Could you check a few things on this model? Use its own coordinates, in mm. Face numbers are marked on the shaded views. A direction names the side the tool comes from. Give positions to 0.01 mm unless a question says otherwise; leave off trailing zeros. Write each loop counter-clockwise with the first axis right and the second up, starting at its lowest first coordinate (ties: lowest second). Pieces come first, ordered by that corner, then holes. Notation, with made-up numbers: (88.5, -26.75) - (122.5, -26.75) arc R21 cw to (122.5, 7.25) - close; hole circle Ø11 at (-40, 57.25). An arc over 180 degrees is marked (long way). Write item = value, one per line.
from build123d import *

# Parameters (mm, degrees)
BOSS_EXTRUDE1_DEPTH = 4
CUT_EXTRUDE2_DEPTH  = 3.25
SKETCH5_W           = 9.5
SKETCH5_H           = 5
BOSS_EXTRUDE2_DEPTH = 8
SKETCH6_W           = 9.5
SKETCH6_H           = 20
BOSS_EXTRUDE3_DEPTH = 3


with BuildPart() as part:
    # Sketch1 → Boss-Extrude1 (new body)
    with BuildSketch(Plane.XY):
        Polygon((0, 0), (40, 40), (-40, 40), align=None)
    extrude(amount=BOSS_EXTRUDE1_DEPTH)

    # Sketch2 → Cut-Extrude2 (cut)
    with BuildSketch(Plane.XY.offset(4)):
        Polygon((0, 2.828427125), (-37.171572875, 40), (-35.757359313, 40), (0, 4.242640687), (35.757359313, 40), (37.171572875, 40), align=None)
    extrude(amount=-CUT_EXTRUDE2_DEPTH, mode=Mode.SUBTRACT)

    # Sketch5 → Boss-Extrude2 (add)
    with BuildSketch(Plane.XY.offset(4)):
        with Locations((0, 24)):
            Rectangle(SKETCH5_W, SKETCH5_H)
    extrude(amount=BOSS_EXTRUDE2_DEPTH)

    # Sketch6 → Boss-Extrude3 (add)
    with BuildSketch(Plane.XY.offset(12)):
        with Locations((0, 31.5)):
            Rectangle(SKETCH6_W, SKETCH6_H)
    extrude(amount=BOSS_EXTRUDE3_DEPTH)


solid = part.part
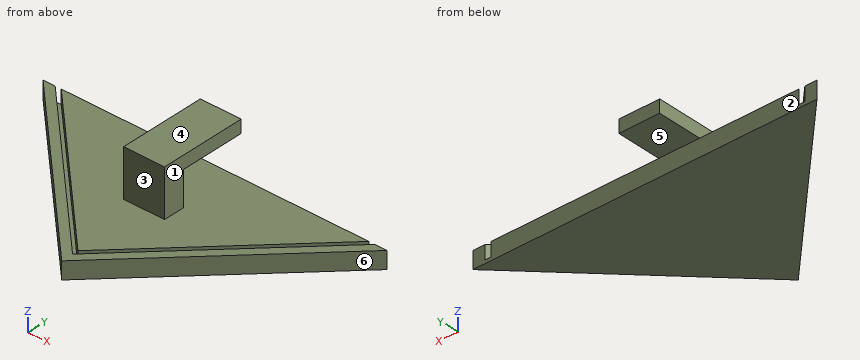
1. For pin 1 (1.2 mm diameter, centred on x = -14.5, z = 2.5, fed in from +Y); pin 2 (1 mm diameter, centred on y = 25.5, z = 2, fed in from +X); pin 3 (3 mm diameter, centred on x = 2, z = 10.5, fed in from -Y); pin 4 (3.5 mm diameter, centred on y = 34, z = 10, fed in from +X), each with a flat end and sliding along its axis, tell me the tip position at first contact or that it passes through.
Filled sheet:
pin_1 = 40
pin_2 = 26
pin_3 = 21.5
pin_4 = through
2. If we section it at C-C, the plane x = -3.5: Please give me the cut outline in (y, z).
Filled sheet:
outline = (3.5, 0) - (40, 0) - (40, 4) - (26.5, 4) - (26.5, 12) - (41.5, 12) - (41.5, 15) - (21.5, 15) - (21.5, 4) - (7.74, 4) - (7.74, 0.75) - (6.33, 0.75) - (6.33, 4) - (3.5, 4) - close
3. I need wall thicknesses on line 1 (Z direction, x = -2.5, y = 38); line 2 (X direction, y = 26, z = 1.75); line 3 (Z direction, x = 18.5, y = 23). Which ranges of each line are inside material? Lowest first, please.
Filled sheet:
line_1 = 0 to 4, 12 to 15
line_2 = -26 to -23.17, -21.76 to 21.76, 23.17 to 26
line_3 = 0 to 4
4. If we section it at A-A, the plane z = 2: Please give me the cut outline in (x, y), and give its area (3 significant figures).
Filled sheet:
outline = (-40, 40) - (0, 0) - (40, 40) - (37.17, 40) - (0, 2.83) - (-37.17, 40) - close; (-35.76, 40) - (0, 4.24) - (35.76, 40) - close
area = 1,500 mm2
5. If we section it at B-B, the plane y = 37: Please give me the cut outline in (x, z), and give its area (3 significant figures).
Filled sheet:
outline = (-37, 0) - (37, 0) - (37, 4) - (34.17, 4) - (34.17, 0.75) - (32.76, 0.75) - (32.76, 4) - (-32.76, 4) - (-32.76, 0.75) - (-34.17, 0.75) - (-34.17, 4) - (-37, 4) - close; (-4.75, 12) - (4.75, 12) - (4.75, 15) - (-4.75, 15) - close
area = 315 mm2
6. Which directions (+Z, -Z, +X, -X, +Y, -Y) give clear straight access to the entire face, cutting with the end or side of a thin tool? Please do the marked faces 1, 2 and 3.
Filled sheet:
face_1 = +Z, +X, +Y, -Y
face_2 = -Z, +X, -X, +Y
face_3 = +Z, +X, -X, -Y
7. If we section it at D-D, the plane y = 25: Please give me the cut outline in (x, z), and give its area (3 significant figures).
Filled sheet:
outline = (-25, 0) - (25, 0) - (25, 4) - (22.17, 4) - (22.17, 0.75) - (20.76, 0.75) - (20.76, 4) - (4.75, 4) - (4.75, 15) - (-4.75, 15) - (-4.75, 4) - (-20.76, 4) - (-20.76, 0.75) - (-22.17, 0.75) - (-22.17, 4) - (-25, 4) - close
area = 295 mm2
8. Thinking about a two-plate mould opening in Z: for the marked faces 4, 5 and 6, which applies, pulls with the +Z half, pulls with the -Z half, needs draft (parallel to the pull), parting line crosses it, or undercut?
Filled sheet:
face_4 = pulls with the +Z half
face_5 = undercut
face_6 = needs draft
